Check sheet for the modelled part. Datum: model origin and axes. Units: mm. A direction names the side the tool comes from. Coordinates: 2 decimals unless noted, no trailing zeros. Write each loop counter-clockwise with the first axis right and the second up, starting at its lowest first coordinate (ties: lowest second). Pieces come first, ordered by that corner, then holes. Notation, with made-up numbers: M -35,76 L -24,76 A17 ccw -24,109 Z; hole C 5.5,86 d9. An arc over 180 degrees is marked long. Answer as CSV lines item,"result". Start each with the question number.
1) Section check D-D (x = 38). Record the cut outline in (y, z), and give its area (3 significant figures).
2) Draft check along Z on faces 1 (the flat face through (2, -3, -27.805)), 2 (the flat face through (-16.687, -3, 4)), 3 (the cylindrical face through (1.555, -1.288, -11.006)). Enter one of: +Z half, -Z half, draft (parallel to the pull), parting line (faces both ways), or undercut.
3) Go/stop test with flat-tipped pins: pin 1 Ø2 at (x, z) = (-0.5, -19.5) entering from +Y; pin 2 Ø0.7 at (x, z) = (17.5, 9.5) entering from +Y; pin 3 Ø3 at (x, y) = (50.5, -1.5) entering from -Z; pin 4 Ø1.5 at (y, z) = (-3.5, -20.5) entering from -X. Record where each tip stops, or that it passes through.
4) Access from +Z, -Z, +X, -X, +Y, -Y to the whole of each face (thin tool, end or side, straight path). Record for faces 4 (the cylindrical face through (15.45, -3.83, -4.36)), 5 (the cylindrical face through (1.805, -1.288, 8.846)), 6 (the flat face through (-39, -3, -2.405)), 7 (the flat face through (43, -3, -15.105)), 8 (the flat face through (21.413, -3, 4)).
5) Section check C-C (z = 1). Record the cut outline in (x, y), and give its area (3 significant figures).
6) Section check B-B (x = 10). Record the cut outline in (y, z).
7) Section check A-A (y = -1.45). Record the cut outline in (x, z), and give its area (3 significant figures).
8) Material ranges on L1, parallel to X at y = -0.4, z = -14.5; L2, parallel to Z at x = 45, y = -3.75; L3, parallel to X at y = -3.4, z = -23, recorded low to high. Write a range as [from, to].
from build123d import *

# Parameters (mm, degrees)
F0_W     = 20.729122051
F0_H     = 12.7
F0_W_2   = 12.7
F0_W_3   = 11.020877949
F0_W_4   = 38.1
F0_W_5   = 44.45
F1_DEPTH = 5.08
F2_R     = 14
F3_DEPTH = 2.54
F4_R     = 1.45
F4_R_2   = 2.5
F5_DEPTH = 25.4


with BuildPart() as f1:
    # F0 (on Front) → F1 (new body)
    with BuildSketch(Plane.XZ):
        with Locations((31.7778353898, -8.7548155423)):
            Rectangle(F0_W, F0_H)
        with Locations((48.4923964153, -8.7548155423)):
            Rectangle(F0_W_2, F0_H)
        with Locations((60.3528353898, -8.7548155423)):
            Rectangle(F0_W_3, F0_H)
        with Locations((2.3632743643, -8.7548155423)):
            Rectangle(F0_W_4, F0_H)
        with Locations((2.3632743643, 3.9451844577)):
            Rectangle(F0_W_4, F0_H)
        with Locations((-38.9117256357, -8.7548155423)):
            Rectangle(F0_W_5, F0_H)
        with Locations((2.3632743643, -21.4548155423)):
            Rectangle(F0_W_4, F0_H)
    extrude(amount=F1_DEPTH)

    # F2 (on face) → F3 (cut)
    with BuildSketch(Plane.XZ.offset(5.08)):
        with Locations((2.0971329576, -8.5653651081)):
            Circle(F2_R)
    extrude(amount=-F3_DEPTH, mode=Mode.SUBTRACT)

    # F4 (on face) → F5 (cut)
    with BuildSketch(Plane.XZ.offset(2.54)):
        with Locations((17.8370033559, 10.2951844577)):
            Circle(F4_R)
        with Locations((1.8370033559, 10.2951844577)):
            Circle(F4_R)
        with Locations((1.8370033559, -14.4356723465)):
            Circle(F4_R)
        with Locations((1.8370033559, 4.5643276535)):
            Circle(F4_R)
        with Locations((2.0971329576, -8.5653651081)):
            Circle(F4_R_2)
    extrude(amount=-F5_DEPTH, mode=Mode.SUBTRACT)


solid = f1.part
Results found:
1,outline,"M -5.08,-15.1 L 0,-15.1 L 0,-2.4 L -5.08,-2.4 Z"
1,area,"64.5 mm2"
2,face 1,"-Z half"
2,face 2,"draft"
2,face 3,"undercut"
3,pin 1,"stops at y = 0"
3,pin 2,"stops at y = -2.54"
3,pin 3,"stops at z = -15.1"
3,pin 4,"stops at x = -16.69"
4,face 4,"-Y"
4,face 5,"+Z, +Y"
4,face 6,"+Z, -X, +Y, -Y"
4,face 7,"-Z, +X, +Y, -Y"
4,face 8,"+Z, +X, +Y, -Y"
5,outline,"M -16.69,-5.08 L -8.13,-5.08 L -8.13,-2.54 L 12.32,-2.54 L 12.32,-5.08 L 21.41,-5.08 L 21.41,0 L -16.69,0 Z"
5,area,"142 mm2"
6,outline,"M -5.08,-27.8 L 0,-27.8 L 0,10.3 L -5.08,10.3 L -5.08,2.99 L -2.54,2.99 L -2.54,-20.12 L -5.08,-20.12 Z"
7,outline,"M -61.14,-15.1 L -16.69,-15.1 L -16.69,-27.8 L 21.41,-27.8 L 21.41,-15.1 L 65.86,-15.1 L 65.86,-2.4 L 21.41,-2.4 L 21.41,10.3 L 19.29,10.3 A1.45 cw 16.39,10.3 L 3.29,10.3 A1.45 cw 0.39,10.3 L -16.69,10.3 L -16.69,-2.4 L -61.14,-2.4 Z; hole C 2.1,-8.57 d5; hole C 1.84,-14.44 d2.9; hole C 1.84,4.56 d2.9"
7,area,"2,540 mm2"
8,L1,"x = [-61.14, 0.39], [3.29, 65.86]"
8,L2,"z = [-15.1, -2.4]"
8,L3,"x = [-16.69, 21.41]"
